The listing builds one solid part. Answer for the finished solid, in the listing's coordinates (mm). Coordinates: 2 decimals unless noted, no trailing zeros. Loops run counter-clockwise (first coordinate to the right, second up) from the corner with the lowest first, then second, coordinate; pieces in that order, holes last. Notation, with made-up numbers: (-37, -34.75) - (-2, -34.75) arc R25 cw to (-2, 4.25) - close; hole circle Ø7 at (-12.75, -10). An arc over 180 degrees is marked (long way). Return JSON: item names as keys, results as strings. Group by question number.
1. Section D-D (x = -0.45) is taken. Write down the section's boundary in (y, z).
2. Each of these flat-tipped pins is pushed along its axis until it touches: P1, Ø1.2, axis at x = 0.79, y = -1.2, coming from the +Z side; P2, Ø1, axis at y = -1, z = 1, coming from the +X side; P3, Ø2.5, axis at y = -1, z = 3.5, coming from the +X side. Where does it stop, or does it pass through?
3. Section C-C (y = 0.1) is taken. Write down the section's boundary in (x, z).
4. Find the intervals of material crossed by line 1 along X through (y, z) = (-1.55, 3.1); line 2 along Z through (x, y) = (1.15, -0.9); line 3 along Z through (x, y) = (-1.2, 1.95), in increasing order.
5. Section B-B (z = 3.05) is taken. Write down the section's boundary in (x, y).
Autodesk Inventor part; units mm, degrees
ref_plane "YZ Plane" through (0, 0, 0) normal (1, 0, 0) x (0, 1, 0)
ref_plane "XZ Plane" through (0, 0, 0) normal (0, 1, 0) x (-1, 0, 0)
ref_plane "XY Plane" through (0, 0, 0) normal (0, 0, 1) x (1, 0, 0)
sketch "Sketch1" plane through (0, 0, 0) normal (0, 0, 1) x (1, 0, 0)
  line L0 (1.75, -2.4) -> (-1.75, -2.4)
  line L1 (-1.75, -2.4) -> (-1.75, 2.4)
  line L2 (-1.75, 2.4) -> (1.75, 2.4)
  line L3 (1.75, 2.4) -> (1.75, -2.4)
  line L4 (1.75, -2.4) -> (-1.75, 2.4) construction
  line L5 (-1.75, -2.4) -> (1.75, 2.4) construction
  point P0 (0, 0)
  dimension "d0" = 3.5
  dimension "d1" = 4.8
extrude "Extrusion1" add sketch "Sketch1" along normal blind 5.1
sketch "Sketch2" plane through (0, 0, 5.1) normal (0, 0, 1) x (1, 0, 0)
  circle A0 centre (0.79, -1.2) radius 0.75
  line L0 (-1.75, 2.4) -> (-1.75, -2.4)
  point P0 (0, 0)
  dimension "d4" = 1.5
  dimension "d5" = 1.2
  dimension "d6" = 2.54
extrude "Extrusion2" cut sketch "Sketch2" against normal blind 0.0254
sketch "Sketch3" plane through (0.79, -1.2, 5.0746) normal (0, 0, 1) x (1, 0, 0)
  circle A0 centre (0, 0) radius 0.75
  line L0 (0.28, -0.75) -> (-0.28, -0.75)
  line L1 (-0.28, -0.75) -> (-0.28, 0.75)
  line L2 (-0.28, 0.75) -> (0.28, 0.75)
  line L3 (0.28, 0.75) -> (0.28, -0.75)
  line L4 (0.28, -0.75) -> (-0.28, 0.75) construction
  line L5 (-0.28, -0.75) -> (0.28, 0.75) construction
  point P0 (-0.79, 1.2)
  point P1 (0, 0.75)
  dimension "d9" = 0.56
extrude "Extrusion3" cut sketch "Sketch3" against normal blind 0.15 contours L3 A0 L1 | A0 L2 L3 | L3 L0 A0 | A0 L1 L2 | L0 L1 A0
sketch "Sketch4" plane through (0, 0, 0) normal (0, 0, -1) x (-1, 0, 0)
  line L0 (-1.95, 1.92) -> (-0.95, 1.92)
  line L1 (-0.95, 1.92) -> (-0.95, 0.62)
  line L2 (-0.95, 0.62) -> (-1.95, 0.62)
  line L3 (-1.95, 0.62) -> (-1.95, 1.92)
  line L4 (-1.95, -0.62) -> (-0.95, -0.62)
  line L5 (-0.95, -0.62) -> (-0.95, -1.92)
  line L6 (-0.95, -1.92) -> (-1.95, -1.92)
  line L7 (-1.95, -1.92) -> (-1.95, -0.62)
  line L8 (0.95, 0.65) -> (1.95, 0.65)
  line L9 (1.95, 0.65) -> (1.95, -0.65)
  line L10 (1.95, -0.65) -> (0.95, -0.65)
  line L11 (0.95, -0.65) -> (0.95, 0.65)
  line L12 (1.75, -2.4) -> (1.75, 2.4)
  line L13 (-1.75, 2.4) -> (-1.75, -2.4)
  line L14 (-1.95, 1.27) -> (-0.95, 1.27) construction
  line L15 (-1.95, -1.27) -> (-0.95, -1.27) construction
  point P0 (0, 0)
  point P1 (0.95, 0)
  dimension "d12" = 1
  dimension "d13" = 1.3
  dimension "d14" = 0.2
  dimension "d15" = 0.2
  dimension "d16" = 2.54
  dimension "d17" = 1.27
extrude "Extrusion4" add sketch "Sketch4" along normal blind 0.2 and the other way blind 0.7
equation "\"d15\" = d14"
properties part number "SM42W"
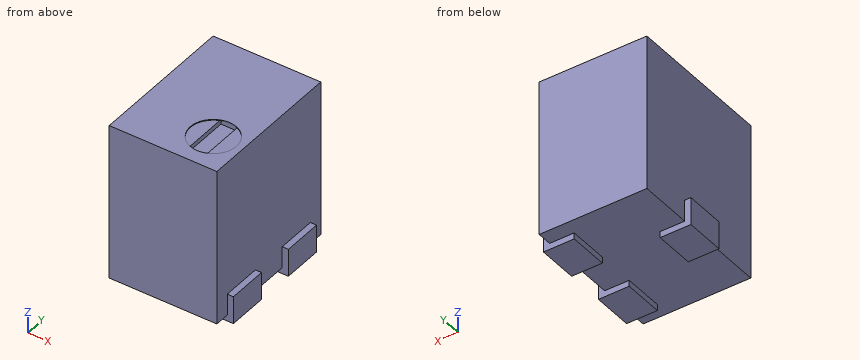
The answers:
{
 "1": {"outline": "(-2.4, 0) - (2.4, 0) - (2.4, 5.1) - (-2.4, 5.1) - close"},
 "2": {"P1": "stops at z = 5.07", "P2": "stops at x = 1.95", "P3": "stops at x = 1.75"},
 "3": {"outline": "(-1.95, -0.2) - (-0.95, -0.2) - (-0.95, 0) - (1.75, 0) - (1.75, 5.1) - (-1.75, 5.1) - (-1.75, 0.7) - (-1.95, 0.7) - close"},
 "4": {"line 1": "x = -1.75 to 1.75", "line 2": "z = -0.2 to 5.07", "line 3": "z = 0 to 5.1"},
 "5": {"outline": "(-1.75, -2.4) - (1.75, -2.4) - (1.75, 2.4) - (-1.75, 2.4) - close"}
}
